```python
from build123d import *

# Parameters (mm, degrees)
SKETCH_1_R             = 6
EXTRUDE_1_DEPTH        = 14
SKETCH_7_R             = 1.6
CUT_EXTRUDE_2_DEPTH    = 32.260998065
HOLE_WIZARD_M3_1_D     = 2.5
HOLE_WIZARD_M3_1_DEPTH = 9.5
HOLE_WIZARD_M3_1_TIP   = 0.751075774


with BuildPart() as part:
    # 草图1 → 凸台-拉伸1 (new, symmetric)
    with BuildSketch(Plane(origin=(0, 0, 0), x_dir=(1, 0, 0), z_dir=(0, 1, 0))):
        with BuildLine():
            Line((-12.5, -25), (12.5, -25))
            Line((12.5, -25), (12.5, 0))
            ThreePointArc((12.5, 0), (0, 12.5), (-12.5, 0))
            Line((-12.5, 0), (-12.5, -25))
        make_face()
        with Locations(Location((0, 0, 0), (0, 0, 270))):
            Circle(SKETCH_1_R, mode=Mode.SUBTRACT)
    extrude(amount=EXTRUDE_1_DEPTH, both=True)

    # 草图7 → 切除-拉伸2 (cut, through all)
    with BuildSketch(Plane.XY):
        with Locations(Location((0, -8, 0), (0, 0, 90))):
            Circle(SKETCH_7_R)
        with Locations(Location((0, 8, 0), (0, 0, 90))):
            Circle(SKETCH_7_R)
    extrude(amount=-CUT_EXTRUDE_2_DEPTH, mode=Mode.SUBTRACT)

    # M3 螺纹孔1
    with Locations(Plane(origin=(-7, -8, 25), x_dir=(1, 0, 0), z_dir=(0, 0, 1))):
        with Locations((0, 0), (14, 0), (14, 16), (0, 16)):
            Hole(HOLE_WIZARD_M3_1_D / 2, depth=HOLE_WIZARD_M3_1_DEPTH)
            with Locations((0, 0, -(HOLE_WIZARD_M3_1_DEPTH + HOLE_WIZARD_M3_1_TIP / 2))):  # 118° drill point
                Cone(0, HOLE_WIZARD_M3_1_D / 2, HOLE_WIZARD_M3_1_TIP, mode=Mode.SUBTRACT)


solid = part.part
```
Geometry: final body of the model. Coordinates: model frame, mm. A direction names the side the tool comes from. Give positions to 0.01 mm unless a question says otherwise; leave off trailing zeros. Order: outer loops, then holes, each group sorted by start corner. A loop starts at its lowest first (then second) coordinate and runs counter-clockwise, first axis right, second up. Notation, with made-up numbers: M 32.25,58 L 91.25,58 A21 cw 91.25,94 Z; hole C -4.75,20.5 d7. An arc over 180 degrees is marked long. Answer as CSV lines item,"result". Start each with the question number.
1) Line query: line 1 (X direction, y = -8, z = 23.25); line 2 (Y direction, x = 7, z = 22.25); line 3 (Z direction, x = -8, y = -3.25). Output: solid intervals per line, ascending. Write a range as from..to.
2) First-contact query: P1, Ø6, axis at y = 6, z = -6, coming from the +X side; P2, Ø3, axis at x = 7, y = -8, coming from the -Z side (3 decimals); P3, Ø8, axis at y = -1, z = -6.5, coming from the -X side. Flat tips, straight axial feed; report the tip coordinate or a pass-through.
3) Mould query, pull axis Y, two halves, no side actions, for faces 4 (the flat face through (0, -14, 10)), 5 (the cylindrical face through (-5.75, 8.05, 20.18)), 6 (the flat face through (12.5, 0, 13)). Classes: +Y half, -Y half, draft (parallel to the pull), parting line (faces both ways), or undercut.
4) Cut plane D-D (y = 3.25). Output: boundary loops of the cut face in (x, z).
5) Cut plane A-A (x = 0). Output: boundary loops of the cut face in (y, z), then the cut area to 3 significant figures.
6) Set-up query: faces 1 (the cylindrical face through (-0.07, 6.4, -9.1)), 2 (the flat face through (0, 14, 10)), 3 (the cylindrical face through (7.99, -8.76, 20.18)). Return all of +Z, -Z, +X, -X, +Y, -Y with unobstructed straight access to the full face (end or side cutting, diameter ignored); none if empty.
7) Cut plane C-C (z = -3). Output: boundary loops of the cut face in (x, y), then the cut area to 3 significant figures.
8) Cut plane B-B (x = -4). Output: boundary loops of the cut face in (y, z).
Findings below:
1,line 1,"x = -12.5..-8.25, -5.75..5.75, 8.25..12.5"
1,line 2,"y = -14..-9.25, -6.75..6.75, 9.25..14"
1,line 3,"z = -9.6..25"
2,P1,"stops at x = 12.13"
2,P2,"stops at z = -11.225"
2,P3,"stops at x = -12.25"
3,face 4,"-Y half"
3,face 5,"undercut"
3,face 6,"draft"
4,outline,"M -12.5,0 A12.5 ccw 12.5,0 L 12.5,25 L -12.5,25 Z; hole C 0,0 d12"
5,outline,"M -14,-12.5 L -9.6,-12.5 L -9.6,-6 L -14,-6 Z; M -14,6 L 14,6 L 14,25 L -14,25 Z; M -6.4,-12.5 L 6.4,-12.5 L 6.4,-6 L -6.4,-6 Z; M 9.6,-12.5 L 14,-12.5 L 14,-6 L 9.6,-6 Z"
5,area,"672 mm²"
6,face 1,"-Z"
6,face 2,"+Z, -Z, +X, -X, +Y"
6,face 3,"+Z"
7,outline,"M -12.13,-14 L -5.2,-14 L -5.2,14 L -12.13,14 Z; M 5.2,-14 L 12.13,-14 L 12.13,14 L 5.2,14 Z"
7,area,"389 mm²"
8,outline,"M -14,-11.84 L 14,-11.84 L 14,-4.47 L -14,-4.47 Z; M -14,4.47 L 14,4.47 L 14,25 L -14,25 Z"
